```python
from build123d import *

# Parameters (mm, degrees)
RESSALTO_EXTRUS_O1_DEPTH = 12.7
CIRCULO_ROLAMENTO_REACH  = 245.52
ESBO_O3_R                = 16
ESBO_O6_R                = 2.5
CORTE_EXTRUS_O4_DEPTH    = 30
CORTE_EXTRUS_O6_REACH    = 245.52
CORTE_EXTRUS_O7_REACH    = 245.52
ESBO_O10_R               = 2.78
CORTE_EXTRUS_O8_REACH    = 245.52
ESBO_O12_R               = 2.78
FILETE1_R                = 10


with BuildPart() as part:
    # Esboço1 → Ressalto-extrusão1 (new body)
    with BuildSketch(Plane.XY):
        Polygon((-114.28595772, -92.023971813), (224.71404228, -92.023971813), (224.71404228, -36.023971813), (5.71404228, -36.023971813), (-54.28595772, 23.976028187), (-54.28595772, 92.976028187), (-114.28595772, 92.976028187), align=None)
    extrude(amount=RESSALTO_EXTRUS_O1_DEPTH)

    # Esboço3 → Circulo rolamento (cut, up to next)
    with BuildSketch(Plane.XY.offset(12.7), mode=Mode.PRIVATE) as circulo_rolamento_sk1:
        with Locations((138.21404228, -64.023971813)):
            Circle(ESBO_O3_R)
    circulo_rolamento_tool1 = extrude(circulo_rolamento_sk1.sketch, amount=-CIRCULO_ROLAMENTO_REACH, mode=Mode.PRIVATE) & part.part
    add(circulo_rolamento_tool1.solids().sort_by_distance((138.214042, -64.023972, 12.7))[0], mode=Mode.SUBTRACT)

    # Esboço6 → Corte-extrusão4 (cut)
    with BuildSketch(Plane.ZY.offset(114.28595772)):
        with Locations(Location((7.9, 67.976028187, 0), (0, 0, 270))):
            Circle(ESBO_O6_R)
        with Locations(Location((7.9, 42.976028187, 0), (0, 0, 270))):
            Circle(ESBO_O6_R)
        with Locations(Location((7.9, 17.976028187, 0), (0, 0, 270))):
            Circle(ESBO_O6_R)
    extrude(amount=-CORTE_EXTRUS_O4_DEPTH, mode=Mode.SUBTRACT)

    # Esboço9 → Corte-extrusão6 (cut, up to next)
    with BuildSketch(Plane.XY.offset(12.7), mode=Mode.PRIVATE) as corte_extrus_o6_sk1:
        Polygon((-29.841868762, -92.023971813), (-114.28595772, -7.579882856), (-114.28595772, -92.023971813), align=None)
    corte_extrus_o6_tool1 = extrude(corte_extrus_o6_sk1.sketch, amount=-CORTE_EXTRUS_O6_REACH, mode=Mode.PRIVATE) & part.part
    add(corte_extrus_o6_tool1.solids().sort_by_distance((-86.137928, -63.875942, 12.7))[0], mode=Mode.SUBTRACT)

    # Esboço10 → Corte-extrusão7 (cut, up to next)
    with BuildSketch(Plane.XY.offset(12.7), mode=Mode.PRIVATE) as corte_extrus_o7_sk1:
        with Locations((56.47404228, -50.023971813)):
            Circle(ESBO_O10_R)
    corte_extrus_o7_tool1 = extrude(corte_extrus_o7_sk1.sketch, amount=-CORTE_EXTRUS_O7_REACH, mode=Mode.PRIVATE) & part.part
    # Esboço10 → Corte-extrusão7 (cut, up to next)
    with BuildSketch(Plane.XY.offset(12.7), mode=Mode.PRIVATE) as corte_extrus_o7_sk2:
        with Locations((56.47404228, -64.023971813)):
            Circle(ESBO_O10_R)
    corte_extrus_o7_tool2 = extrude(corte_extrus_o7_sk2.sketch, amount=-CORTE_EXTRUS_O7_REACH, mode=Mode.PRIVATE) & part.part
    # Esboço10 → Corte-extrusão7 (cut, up to next)
    with BuildSketch(Plane.XY.offset(12.7), mode=Mode.PRIVATE) as corte_extrus_o7_sk3:
        with Locations((56.47404228, -78.023971813)):
            Circle(ESBO_O10_R)
    corte_extrus_o7_tool3 = extrude(corte_extrus_o7_sk3.sketch, amount=-CORTE_EXTRUS_O7_REACH, mode=Mode.PRIVATE) & part.part
    add(corte_extrus_o7_tool1.solids().sort_by_distance((56.474042, -50.023972, 12.7))[0], mode=Mode.SUBTRACT)
    add(corte_extrus_o7_tool2.solids().sort_by_distance((56.474042, -64.023972, 12.7))[0], mode=Mode.SUBTRACT)
    add(corte_extrus_o7_tool3.solids().sort_by_distance((56.474042, -78.023972, 12.7))[0], mode=Mode.SUBTRACT)

    # Esboço12 → Corte-extrusão8 (cut, up to next)
    with BuildSketch(Plane.XY.offset(12.7), mode=Mode.PRIVATE) as corte_extrus_o8_sk1:
        with Locations((219.95404228, -78.023971813)):
            Circle(ESBO_O12_R)
    corte_extrus_o8_tool1 = extrude(corte_extrus_o8_sk1.sketch, amount=-CORTE_EXTRUS_O8_REACH, mode=Mode.PRIVATE) & part.part
    # Esboço12 → Corte-extrusão8 (cut, up to next)
    with BuildSketch(Plane.XY.offset(12.7), mode=Mode.PRIVATE) as corte_extrus_o8_sk2:
        with Locations((219.95404228, -64.023971813)):
            Circle(ESBO_O12_R)
    corte_extrus_o8_tool2 = extrude(corte_extrus_o8_sk2.sketch, amount=-CORTE_EXTRUS_O8_REACH, mode=Mode.PRIVATE) & part.part
    # Esboço12 → Corte-extrusão8 (cut, up to next)
    with BuildSketch(Plane.XY.offset(12.7), mode=Mode.PRIVATE) as corte_extrus_o8_sk3:
        with Locations((219.95404228, -50.023971813)):
            Circle(ESBO_O12_R)
    corte_extrus_o8_tool3 = extrude(corte_extrus_o8_sk3.sketch, amount=-CORTE_EXTRUS_O8_REACH, mode=Mode.PRIVATE) & part.part
    add(corte_extrus_o8_tool1.solids().sort_by_distance((219.954042, -78.023972, 12.7))[0], mode=Mode.SUBTRACT)
    add(corte_extrus_o8_tool2.solids().sort_by_distance((219.954042, -64.023972, 12.7))[0], mode=Mode.SUBTRACT)
    add(corte_extrus_o8_tool3.solids().sort_by_distance((219.954042, -50.023972, 12.7))[0], mode=Mode.SUBTRACT)

    # Filete1
    filete1_edges = [part.edges().sort_by_distance(p)[0] for p in [
        (-54.28595772, 92.976028187, 6.35),
        (-54.28595772, 23.976028187, 6.35),
        (5.71404228, -36.023971813, 6.35),
        (-29.841868762, -92.023971813, 6.35),
    ]]
    fillet(filete1_edges, radius=FILETE1_R)


solid = part.part
```
Verification items for the finished model (mm, model axes). A direction names the side the tool comes from. Give positions to 0.01 mm unless a question says otherwise; leave off trailing zeros. Write each loop counter-clockwise with the first axis right and the second up, starting at its lowest first coordinate (ties: lowest second). Pieces come first, ordered by that corner, then holes. Notation, with made-up numbers: M -33,-35.75 L -8,-35.75 A32 ccw -8,-2.75 Z; hole C -36,7 d10. An arc over 180 degrees is marked long. One line per question, with ' | ' between items.
1) Thickness scan on line 1 along Z through (x, y) = (-89.5, 42.5); line 2 along Y through (x, z) = (175, 11); line 3 along X through (y, z) = (68.5, 8). Record the ranges inside material, lowest first. Write a range as [from, to].
Result:
line 1: z = [0, 5.45], [10.35, 12.7] | line 2: y = [-92.02, -36.02] | line 3: x = [-84.29, -54.29]
2) Mould release check, pull along X, two halves, no side actions. Record for faces 1 (the cylindrical face through (-57.29, 90.12, 6.44)), 2 (the flat face through (-89, 92.976, 6)), 3 (the cylindrical face through (153.475, -59.218, 6.439)), 4 (the cylindrical face through (-29.48, -91.28, 6.26)): released by +X, released by -X, zero draft, split by the parting line, or undercut.
Result:
face 1: released by +X | face 2: zero draft | face 3: undercut | face 4: released by -X
3) Section check D-D on y = -23.5. Enter the section's corners in (x, z), plus the area to 3 significant figures.
Result:
outline: M -98.37,0 L -6.81,0 L -6.81,12.7 L -98.37,12.7 Z | area: 1,160 mm2
4) Gauge pin test, flat ends, axial feed: pin 1 Ø1 at (x, z) = (-38, 6) entering from -Y; pin 2 Ø3 at (y, z) = (17.98, 7.9) entering from -X; pin 3 Ø3.5 at (x, y) = (56.47, -78.02) entering from -Z; pin 4 Ø4.5 at (y, z) = (67.98, 7.9) entering from +X. Record the tip position at first contact, or that the pin passes through.
Result:
pin 1: stops at y = -84.37 | pin 2: stops at x = -84.29 | pin 3: passes through | pin 4: stops at x = -54.29
5) Section check A-A on z = 7.9. State how many separate pieces and enclosed holes the cut face has, plus the area to 3 significant figures.
Result:
separate pieces: 1 | enclosed holes: 7 | area: 23,500 mm2
6) Set-up check for faces 5 (the flat face through (-54.286, 55, 6)), 6 (the flat face through (98, -92.024, 6)): record each of +Z, -Z, +X, -X, +Y, -Y from which the full face is reachable in a straight line by a thin tool's end or side.
Result:
face 5: +Z, -Z, +X, +Y | face 6: +Z, -Z, +X, -X, -Y
7) Section check C-C on x = -48. Enter the section's corners in (y, z).
Result:
outline: M -73.87,0 L 17.69,0 L 17.69,12.7 L -73.87,12.7 Z
8) Section check B-B on x = 140. Enter the section's corners in (y, z).
Result:
outline: M -92.02,0 L -79.92,0 L -79.92,12.7 L -92.02,12.7 Z; M -48.12,0 L -36.02,0 L -36.02,12.7 L -48.12,12.7 Z
